Job drawing, mm, ordinate dimensions from the low corner. One solid piece. A direction names the side the tool comes from. Give positions to 0.01 mm unless a question says otherwise; leave off trailing zeros. Order: outer loops, then holes, each group sorted by start corner. A loop starts at its lowest first (then second) coordinate and runs counter-clockwise, first axis right, second up. Notation, with made-up numbers: (-8, -24.5) - (-2, -24.5) arc R28 ccw to (-2, -6.5) - close; hole circle Ø2 at (-2, 21). An arc over 180 degrees is marked (long way). One line per item, written item: value.
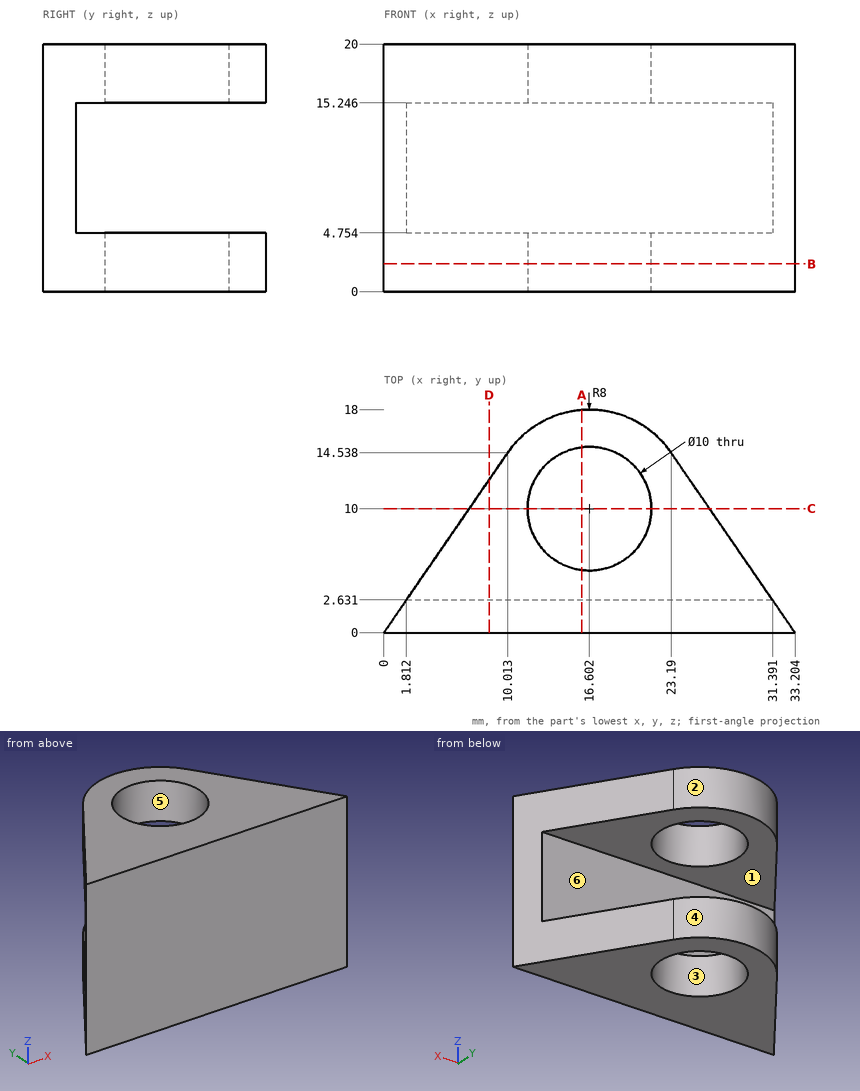
1) Slice it at A-A on x = 16. Write the cut outline in (y, z) (1 decimal), then the cut area to 3 significant figures.
Answer:
outline: (0, 0) - (5, 0) - (5, 4.8) - (2.6, 4.8) - (2.6, 15.2) - (5, 15.2) - (5, 20) - (0, 20) - close; (15, 0) - (18, 0) - (18, 4.8) - (15, 4.8) - close; (15, 15.2) - (18, 15.2) - (18, 20) - (15, 20) - close
area: 104 mm2
2) Which spindle directions (+Z, -Z, +X, -X, +Y, -Y) get a long thin tool onto all of the face, cutting with end or side? Do the marked faces 1 and 2. Say none if no direction does.
Answer:
face 1: +X, -X, +Y
face 2: +Z, -Z, +Y
3) Wall check: line 1 along Z through (x, y) = (23.5, 11.75) (1 decimal); line 2 along Y through (x, z) = (19.5, 14.75); line 3 along Y through (x, z) = (15.5, 2.75). Give the ranges that are in metal, low to high. Write a range as [from, to].
Answer:
line 1: z = [0, 4.8], [15.2, 20]
line 2: y = [0, 2.63]
line 3: y = [0, 5.12], [14.88, 17.92]
4) Slice it at B-B on z = 2.25. Write the cut outline in (x, y).
Answer:
outline: (0, 0) - (33.2, 0) - (23.19, 14.54) arc R8 ccw to (10.01, 14.54) - close; hole circle Ø10 at (16.6, 10)
5) Two-plate mould, pull along X, no slides. Class the marked faces 3, 4, 5 and 6: pulls with the +X half, pulls with the -X half, needs draft (parallel to the pull), parting line crosses it, or undercut.
Answer:
face 3: undercut
face 4: parting line crosses it
face 5: undercut
face 6: needs draft
6) Drop flat-ended pins along their axis: P1, Ø1, axis at y = 8, z = 13, coming from the -X side; P2, Ø6, axis at y = 9.5, z = 14, coming from the +X side; P3, Ø2, axis at y = 15.5, z = 17.5, coming from the +X side; P4, Ø5, axis at x = 15, z = 10, coming from the +Y side. Give the stop position or say it passes through.
Answer:
P1: passes through
P2: stops at x = 28.54
P3: stops at x = 23.22
P4: stops at y = 2.63
7) Slice it at C-C on y = 10. Write the cut outline in (x, z) (1 decimal).
Answer:
outline: (6.9, 0) - (11.6, 0) - (11.6, 4.8) - (6.9, 4.8) - close; (6.9, 15.2) - (11.6, 15.2) - (11.6, 20) - (6.9, 20) - close; (21.6, 0) - (26.3, 0) - (26.3, 4.8) - (21.6, 4.8) - close; (21.6, 15.2) - (26.3, 15.2) - (26.3, 20) - (21.6, 20) - close
8) Slice it at D-D on x = 8.5. Write the cut outline in (y, z) (1 decimal).
Answer:
outline: (0, 0) - (12.3, 0) - (12.3, 4.8) - (2.6, 4.8) - (2.6, 15.2) - (12.3, 15.2) - (12.3, 20) - (0, 20) - close
